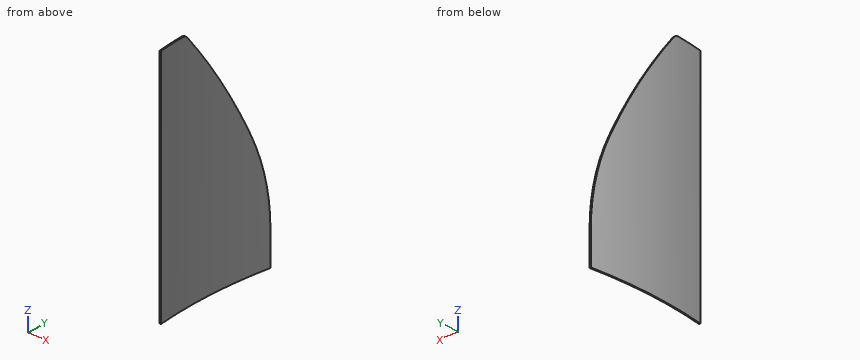
```python
from build123d import *

# Parameters (mm, degrees)
EXTRUDE_THIN1_DEPTH = 500
SKETCH2_OUTSIDE_W   = 1225.724
SKETCH2_OUTSIDE_H   = 726.468
CUT_EXTRUDE1_DEPTH  = 40
CUT_EXTRUDE2_DEPTH  = 905.0000001


with BuildPart() as part:
    # Sketch1 → Extrude-Thin1 (new body, symmetric)
    with BuildSketch(Plane.XY):
        with BuildLine():
            ThreePointArc((2.472217938, 0.371669838), (-16.187326406, 250), (2.472217938, 499.628330162))
            Line((2.472217938, 499.628330162), (-2.472217938, 500.371669838))
            ThreePointArc((-2.472217938, 500.371669838), (-21.187326406, 250), (-2.472217938, -0.371669838))
            Line((-2.472217938, -0.371669838), (2.472217938, 0.371669838))
        make_face()
    extrude(amount=EXTRUDE_THIN1_DEPTH, both=True)

    # Sketch2 outside → Cut-Extrude1 (cut, symmetric)
    with BuildSketch(Plane(origin=(0, 0, 0), x_dir=(0, 0, -1), z_dir=(1, 0, 0))):
        with Locations((0, 250)):
            Rectangle(SKETCH2_OUTSIDE_W, SKETCH2_OUTSIDE_H)
        with BuildLine():
            Line((500, 499.628330162), (370, 499.628330162))
            ThreePointArc((370, 499.628330162), (198.298251655, 480.98516901), (34.59916172, 425.9246042))
            ThreePointArc((34.59916172, 425.9246042), (-187.662872816, 305.701379942), (-392.991389707, 158.411747589))
            ThreePointArc((-392.991389707, 158.411747589), (-401.108501353, 148.038589085), (-404, 135.188330162))
            Line((-404, 135.188330162), (-404, 30.188330162))
            Line((-404, 30.188330162), (500, 30.188330162))
            Line((500, 30.188330162), (500, 499.628330162))
        make_face(mode=Mode.SUBTRACT)
    extrude(amount=CUT_EXTRUDE1_DEPTH, both=True, mode=Mode.SUBTRACT)

    # Sketch3 → Cut-Extrude2 (cut, through all)
    with BuildSketch(Plane.XY.offset(404)):
        Polygon((-6.780603569, 30.188330162), (-1.858216297, 31.105746602), (-1.737331603, 30.188330162), align=None)
    extrude(amount=-CUT_EXTRUDE2_DEPTH, mode=Mode.SUBTRACT)


solid = part.part
```
The model under review builds one solid part; all positions refer to its coordinate system, in mm. Give positions to 0.01 mm unless a question says otherwise; leave off trailing zeros. Write each loop counter-clockwise with the first axis right and the second up, starting at its lowest first coordinate (ties: lowest second). Pieces come first, ordered by that corner, then holes.
(1) For P1, Ø8, axis at y = 347.5, z = -3, coming from the -X side; P2, Ø10, axis at y = 199.5, z = 256, coming from the +X side, all flat-tipped, find the tip position at first contact; note any pin that passes through.
(2) Consider section A-A, the plane y = 98. Give the boundary of the cut face in (x, z).
(3) To check wall thickness, follow L1, parallel to X at y = 362, z = -153.5; L2, parallel to X at y = 232.5, z = -379.5; L3, parallel to Z at x = -16.25, y = 188.5. State the ranges of each line that lie inside material, in increasing order.
(4) Consider section B-B, the plane z = 235. Give the boundary of the cut face in (x, y).
Returned:
1. P1: stops at x = -18.59
1. P2: stops at x = -15.27
2. outline: (-14.31, -500) - (-9.29, -500) - (-9.29, 404) - (-14.31, 404) - close
3. L1: x = -17.46 to -12.45
3. L2: x = -21.1 to -16.1
3. L3: z = -500 to 355.28
4. outline: (-21, 275.15) arc R1684.1 ccw to (-6.78, 30.19) - (-1.86, 31.11) arc R1679.1 cw to (-16, 275.15) - close
